Build history of the part. All positions in model axes, mm. A direction names the side the tool comes from. Give positions to 0.01 mm unless a question says otherwise; leave off trailing zeros. Order: outer loops, then holes, each group sorted by start corner. A loop starts at its lowest first (then second) coordinate and runs counter-clockwise, first axis right, second up. Notation, with made-up numbers: (-27, 56.5) - (-14, 56.5) arc R12 ccw to (-14, 65.5) - close; hole circle Ø7 at (3.25, 14). An arc over 180 degrees is marked (long way). Use a Markdown table: item, result. Add a question column.
(1) Slice it at A-A (z = 126). Write the cut outline in (x, y).
(2) Wall check: line 1 (X direction, y = -43, z = 114); line 2 (X direction, y = -42.75, z = 114.3); line 3 (Y direction, x = 2, z = -33). Give the ranges that are in metal, low to high.
(3) Mould opens along X. For faces 5 (the face through (-37.13, 59.501, -18.706)), 6 (the face through (-34.88, 58.2, 114.76)), 7 (the face through (35, -3, 0)), 8 (the face through (-11.913, 48.557, 43.116)) say: +X half, -X half, draft (parallel to the pull), parting line (faces both ways), or undercut.
(4) Slice it at C-C (z = 32). Write the cut outline in (x, y).
(5) Flat gauge pins, fed straight in: pin 1 (12 mm diameter, centred on x = 6.5, z = 68, fed in from +Y); pin 2 (7 mm diameter, centred on x = 56, y = -42.5, fed in from +Z); pin 3 (6 mm diameter, centred on x = 22, z = 85.5, fed in from +Y); pin 4 (4 mm diameter, centred on x = 33, y = -24, fed in from -Z). Where does each tip first touch, or does it go through?
(6) Slice it at B-B (y = 44). Write the cut outline in (x, z), then the cut area to 3 significant figures.
(7) Which spindle directions (+Z, -Z, +X, -X, +Y, -Y) get a long thin tool onto all of the face, cutting with end or side? Do faces 1 (the face through (29.855, 20.725, 43.117)), 2 (the face through (35, -3, 88.9)), 3 (the face through (37, -43, 133.35)), 4 (the face through (37, -43, -44.45)). Say none if no direction does.
(8) Slice it at D-D (x = 66.5). Write the cut outline in (y, z), then the cut area to 3 significant figures.
Autodesk Inventor part; units mm, degrees
ref_plane "YZ Plane" through (0, 0, 0) normal (1, 0, 0) x (0, 1, 0)
ref_plane "XZ Plane" through (0, 0, 0) normal (0, 1, 0) x (-1, 0, 0)
ref_plane "XY Plane" through (0, 0, 0) normal (0, 0, 1) x (1, 0, 0)
sketch "Sketch1" plane through (0, 0, 0) normal (0, 0, 1) x (1, 0, 0)
  line L0 (28.2901, 18.0136) -> (77.2705, -40.359)
  line L1 (77.2705, -40.359) -> (51.8705, -40.359)
  line L2 (51.8705, -40.359) -> (-20.9781, 46.4586)
  line L3 (-20.9781, 46.4586) -> (28.2901, 18.0136)
  point P0 (0, 0)
  point P1 (3.656, 32.2361)
  dimension "d0" = 76.2
  dimension "d2" = 25.4
  dimension "d34" = 130
  dimension "d35" = 160
extrude "Extrusion1" add sketch "Sketch1" along normal blind 88.9
sketch "Sketch2" plane through (-20.9781, 46.4586, 0) normal (0.5, 0.8660254, 0) x (0, 0, 1)
  line L0 (0, 0) -> (0, 56.89)
  line L1 (-50.8, 56.89) -> (139.7, 56.89)
  line L2 (139.7, 56.89) -> (139.7, -44.71)
  line L3 (139.7, -44.71) -> (-50.8, -44.71)
  line L4 (-50.8, -44.71) -> (-50.8, 56.89)
  line L5 (0, 56.89) -> (88.9, 56.89)
  point P0 (0, 41.3969)
  point P1 (44.45, 19.4575)
  dimension "d6" = 190.5
  dimension "d8" = 95.25
  dimension "d9" = 101.6
  dimension "d10" = 44.45
  dimension "d11" = 88.9
  dimension "d12" = 56.89
  dimension "d45" = 0
extrude "Extrusion2" add sketch "Sketch2" along normal blind 6.35
sketch "Sketch3" plane through (-17.8031, 51.9578, 0) normal (0.5, 0.8660254, 0) x (0, 0, 1)
  line L0 (139.7, 56.89) -> (-50.8, 56.89)
  circle A0 centre (-22.225, -19.05) radius 3.81
  circle A1 centre (111.125, -19.05) radius 3.81
  line L1 (-50.8, -44.71) -> (139.7, -44.71)
  line L2 (44.45, -44.71) -> (44.45, 56.89)
  line L3 (0, 0) -> (88.9, 0)
  point P0 (0, 41.3969)
  dimension "d17" = 7.62
  dimension "d18" = 7.62
  dimension "d19" = 0
  dimension "d46" = 133.35
  dimension "d47" = 66.675
  dimension "d86" = 19.05
extrude "Extrusion3" cut sketch "Sketch3" against normal up to next
sketch "Sketch6" plane through (-17.8031, 51.9578, 0) normal (0.5, 0.8660254, 0) x (0.8660254, -0.5, 0)
  circle A0 centre (-19.05, 22.225) radius 3.81
  circle A1 centre (-19.05, -111.125) radius 3.81
  line L0 (6.35, 34.925) -> (-44.45, 34.925)
  line L1 (-44.45, 34.925) -> (-44.45, -15.875)
  line L2 (-44.45, -15.875) -> (6.35, -15.875)
  line L3 (6.35, -15.875) -> (6.35, 34.925)
  line L4 (6.35, -73.025) -> (-44.45, -73.025)
  line L5 (-44.45, -73.025) -> (-44.45, -123.825)
  line L6 (-44.45, -123.825) -> (6.35, -123.825)
  line L7 (6.35, -123.825) -> (6.35, -73.025)
  point P0 (41.3969, 0)
  dimension "d52" = 50.8
  dimension "d60" = 25.4
  dimension "d61" = 25.4
  dimension "d62" = 50.8
  dimension "d63" = 12.7
  dimension "d64" = 12.7
extrude "Extrusion5" [suppressed]
sketch "Sketch7" plane through (-18.1206, 51.4079, 0) normal (0.5, 0.8660254, 0) x (0.8660254, -0.5, 0)
  line L0 (6.35, 38.1) -> (-44.45, 38.1)
  line L1 (6.35, -76.2) -> (-44.45, -76.2)
  line L2 (-44.45, -76.2) -> (-44.45, -127)
  line L3 (-44.45, -127) -> (6.35, -127)
  line L4 (6.35, -127) -> (6.35, -76.2)
  line L5 (-44.45, -12.7) -> (-39.2324, -12.7)
  line L6 (-39.2324, -12.7) -> (-39.2324, 38.1)
  line L7 (-39.2324, 38.1) -> (-44.45, 38.1)
  line L8 (-44.45, 38.1) -> (-44.45, -12.7)
  line L9 (-44.45, -127) -> (-39.2324, -127)
  line L10 (-39.2324, -127) -> (-39.2324, -76.2)
  line L11 (-39.2324, -76.2) -> (-44.45, -76.2)
  line L12 (-44.45, -76.2) -> (-44.45, -127)
  point P0 (41.3969, 0)
  dimension "d56" = 5.2176
  dimension "d57" = 5.2176
extrude "Extrusion6" [suppressed]
sketch "Sketch13" plane through (-57.8855, 71.4332, -38.1) normal (-0.8660254, 0.5, 0) x (0, 0, 1)
  line L0 (0, 0) -> (0, 2.54)
  circle A0 centre (25.4, 39.096) radius 3.175
  circle A1 centre (139.7, 39.096) radius 3.175
  line L1 (114.3, 0) -> (114.3, 2.54)
  point P0 (50.8, 53.34)
  point P1 (0, 53.34)
  point P2 (38.1, -32.9202)
  point P3 (114.3, 53.34)
  dimension "d98" = 6.35
  dimension "d99" = 0
  dimension "d100" = 25.4
  dimension "d101" = 50.8
  dimension "d102" = 25.4
extrude "Extrusion11" [suppressed]
sketch "Sketch14" plane through (-57.8855, 71.4332, -38.1) normal (-0.8660254, 0.5, 0) x (0, 0, 1)
  circle A0 centre (25.4, 39.096) radius 3.175
  line L0 (-107.95, 213.721) -> (273.05, 213.721)
  line L1 (273.05, 213.721) -> (273.05, -14.879)
  line L2 (273.05, -14.879) -> (-107.95, -14.879)
  line L3 (-107.95, -14.879) -> (-107.95, 213.721)
  point P0 (38.1, -32.9202)
  dimension "d107" = 381
  dimension "d109" = 228.6
  dimension "d110" = 133.35
  dimension "d111" = 53.975
extrude "Extrusion12" [suppressed]
sketch "Sketch18" plane through (-57.8855, 71.4332, -38.1) normal (0.8660254, -0.5, 0) x (0, 0, -1)
  line L0 (-273.05, -14.879) -> (107.95, -14.879)
  line L1 (-273.05, 213.721) -> (-195.9898, 213.721)
  line L2 (-195.9898, 213.721) -> (-195.9898, -14.879)
  line L3 (-195.9898, -14.879) -> (-273.05, -14.879)
  line L4 (-273.05, -14.879) -> (-273.05, 213.721)
  line L5 (107.95, 213.721) -> (30.8898, 213.721)
  line L6 (30.8898, 213.721) -> (30.8898, -14.879)
  line L7 (30.8898, -14.879) -> (107.95, -14.879)
  line L8 (107.95, -14.879) -> (107.95, 213.721)
  point P0 (-38.1, -32.9202)
extrude "Extrusion14" [suppressed]
sketch "Sketch15" plane through (0, 0, 0) normal (0, 0, 1) x (1, 0, 0)
  line L0 (15.9795, 275.571) -> (4.9809, 281.921)
  line L1 (-109.3191, 83.9476) -> (4.9809, 281.921)
  line L2 (-98.3205, 77.5976) -> (-109.3191, 83.9476)
  line L3 (77.2705, -40.359) -> (28.2901, 18.0136)
  line L4 (28.2901, 18.0136) -> (-20.9781, 46.4586)
  line L5 (-20.9781, 46.4586) -> (51.8705, -40.359)
  line L6 (51.8705, -40.359) -> (77.2705, -40.359)
  line L7 (77.2705, -40.359) -> (-405.3295, -40.359)
  line L8 (77.2705, -40.359) -> (204.2705, -40.359)
  line L9 (-98.3205, 77.5976) -> (15.9795, 275.571)
  point P0 (0, 0)
  point P1 (-65.325, 58.5476)
  point P2 (48.975, 256.521)
  dimension "d125" = 127
  dimension "d127" = 482.6
sketch "Sketch16" plane through (0, 0, 0) normal (0, 0, 1) x (1, 0, 0)
  line L0 (77.2705, -40.359) -> (-405.3295, -40.359)
  line L1 (15.9795, 275.571) -> (4.9809, 281.921)
  line L2 (-109.3191, 83.9476) -> (4.9809, 281.921)
  line L3 (-98.3205, 77.5976) -> (-109.3191, 83.9476)
  line L4 (77.2705, -40.359) -> (204.2705, -40.359)
  line L5 (-98.3205, 77.5976) -> (15.9795, 275.571)
  point P0 (0, 0)
  point P1 (-65.325, 58.5476)
  point P2 (51.8705, -40.359)
  point P3 (51.8705, -40.359)
  dimension "d129" = 457.2
  dimension "d130" = 322.28
  dimension "d131" = 98.9066
  dimension "d150" = 188.291
sketch "Sketch17" plane through (0, 0, 0) normal (0, 0, 1) x (1, 0, 0)
  line L0 (77.2705, -40.359) -> (-405.3295, -40.359)
  line L1 (-144.0325, 61.241) -> (-144.0325, -40.359)
  line L2 (-144.0325, -40.359) -> (-42.4325, -40.359)
  line L3 (-42.4325, -40.359) -> (-42.4325, 35.841)
  line L4 (-42.4325, 35.841) -> (-144.0325, 61.241)
  line L5 (77.2705, -40.359) -> (204.2705, -40.359)
  point P0 (0, 0)
  point P1 (-93.2325, -40.359)
  dimension "d141" = 101.6
  dimension "d142" = 101.6
  dimension "d146" = 76.2
  dimension "d147" = 297.503
  dimension "d151" = 312.097
extrude "Extrusion13" [suppressed]
sketch "Sketch19" plane through (51.8705, -40.359, 0) normal (0, -1, 0) x (1, 0, 0)
  line L0 (25.4, 0) -> (0, 0)
  line L1 (25.4, 0) -> (25.4, 88.9)
  line L2 (0, 88.9) -> (25.4, 88.9)
  line L3 (0, 0) -> (0, 88.9)
  line L4 (25.4, 88.9) -> (25.4, 133.35)
  line L5 (25.4, 133.35) -> (-56.7156, 133.35)
  line L6 (-56.7156, 133.35) -> (-56.7156, 71.7364)
  line L7 (25.4, 0) -> (25.4, -44.45)
  line L8 (25.4, -44.45) -> (-56.7156, -44.45)
  line L9 (-56.7156, -44.45) -> (-56.7156, 17.1636)
  line L10 (-56.7156, 71.7364) -> (-56.7156, 17.1636)
  point P0 (-51.8705, 0)
  dimension "d153" = 90
  dimension "d155" = 90
  dimension "d156" = 90
  dimension "d159" = 90
  dimension "d160" = 44.45
extrude "Extrusion15" add sketch "Sketch19" along normal blind 6.35
sketch "Sketch20" plane through (51.8705, -40.359, 0) normal (0, 1, 0) x (1, 0, 0)
  line L0 (25.4, 44.45) -> (25.4, 0)
  line L1 (-56.7156, 44.45) -> (25.4, 44.45)
  line L2 (25.4, -133.35) -> (-56.7156, -133.35)
  line L3 (25.4, -88.9) -> (25.4, -133.35)
  circle A0 centre (0, 25.4) radius 1.5875
  circle A1 centre (0, -114.3) radius 1.5875
  point P0 (-51.8705, 0)
  dimension "d161" = 3.175
  dimension "d162" = 19.05
  dimension "d163" = 25.4
  dimension "d164" = 19.05
  dimension "d165" = 25.4
extrude "Extrusion16" cut sketch "Sketch20" against normal blind 6.35
sketch "Sketch21" plane through (51.8705, -46.709, 0) normal (0, -1, 0) x (1, 0, 0)
  line L0 (25.4, 133.35) -> (-56.7156, 133.35)
  line L1 (-56.7156, -44.45) -> (25.4, -44.45)
  line L2 (23.5667, 45.085) -> (31.1867, 45.085)
  line L3 (31.1867, 45.085) -> (31.1867, 43.815)
  line L4 (31.1867, 43.815) -> (23.5667, 43.815)
  line L5 (23.5667, 43.815) -> (23.5667, 45.085)
  point P0 (-51.8705, 0)
  dimension "d168" = 1.27
  dimension "d170" = 177.8
  dimension "d171" = 88.265
  dimension "d172" = 7.62
extrude "Extrusion17" cut sketch "Sketch21" against normal blind 25.4
equation "\"d18\" = d17"
equation "\"d47\" = 0.5 * d46"
equation "\"d61\" = d60"
equation "\"d64\" = d63"
equation "\"d57\" = d56"
equation "\"d100\" = 0.5 * d101"
equation "\"d102\" = d100"
equation "\"d156\" = d155"
equation "\"d164\" = d162"
equation "\"d165\" = d163"
equation "\"d171\" = 0.5 * d170 - 0.5 * d168"
properties part number "Problem Solving"
Solution:
| question | item | result |
|---|---|---|
| 1 | outline | (-59.7, 68.81) - (28.29, 18.01) - (31.47, 23.51) - (-56.52, 74.31) - close; (-4.85, -46.71) - (77.27, -46.71) - (77.27, -40.36) - (-4.85, -40.36) - close |
| 2 | line 1 | -4.85 to 50.31, 53.43 to 77.27 |
| 2 | line 2 | -4.85 to 50.28, 53.46 to 77.27 |
| 2 | line 3 | -46.71 to -40.36, 33.19 to 40.52 |
| 3 | face 5 | undercut |
| 3 | face 6 | undercut |
| 3 | face 7 | draft |
| 3 | face 8 | +X half |
| 4 | outline | (-59.7, 68.81) - (-20.98, 46.46) - (51.87, -40.36) - (-4.85, -40.36) - (-4.85, -46.71) - (77.27, -46.71) - (77.27, -40.36) - (28.29, 18.01) - (31.47, 23.51) - (-56.52, 74.31) - close |
| 5 | pin 1 | y = 41.39 |
| 5 | pin 2 | z = 133.35 |
| 5 | pin 3 | y = 30.71 |
| 5 | pin 4 | through |
| 6 | outline | (-18.92, 0) - (-16.72, 0) - (-16.72, -50.8) - (-4.02, -50.8) - (-4.02, 139.7) - (-16.72, 139.7) - (-16.72, 88.9) - (-18.92, 88.9) - close |
| 6 | area | 2,610 mm2 |
| 7 | face 1 | +Z, -Z, +X |
| 7 | face 2 | +Z, -X |
| 7 | face 3 | +Z, +X, -X, -Y |
| 7 | face 4 | -Z, +X, -X, -Y |
| 8 | outline | (-46.71, -44.45) - (-40.36, -44.45) - (-40.36, 0) - (-27.52, 0) - (-27.52, 88.9) - (-40.36, 88.9) - (-40.36, 133.35) - (-46.71, 133.35) - close |
| 8 | area | 2,270 mm2 |
